Drawing for the job (mm, zero at the part's lowest x, y, z). Give positions to 0.01 mm unless a question says otherwise; leave off trailing zeros. Answer as a JSON object with one key per item and string values. Group by question number.
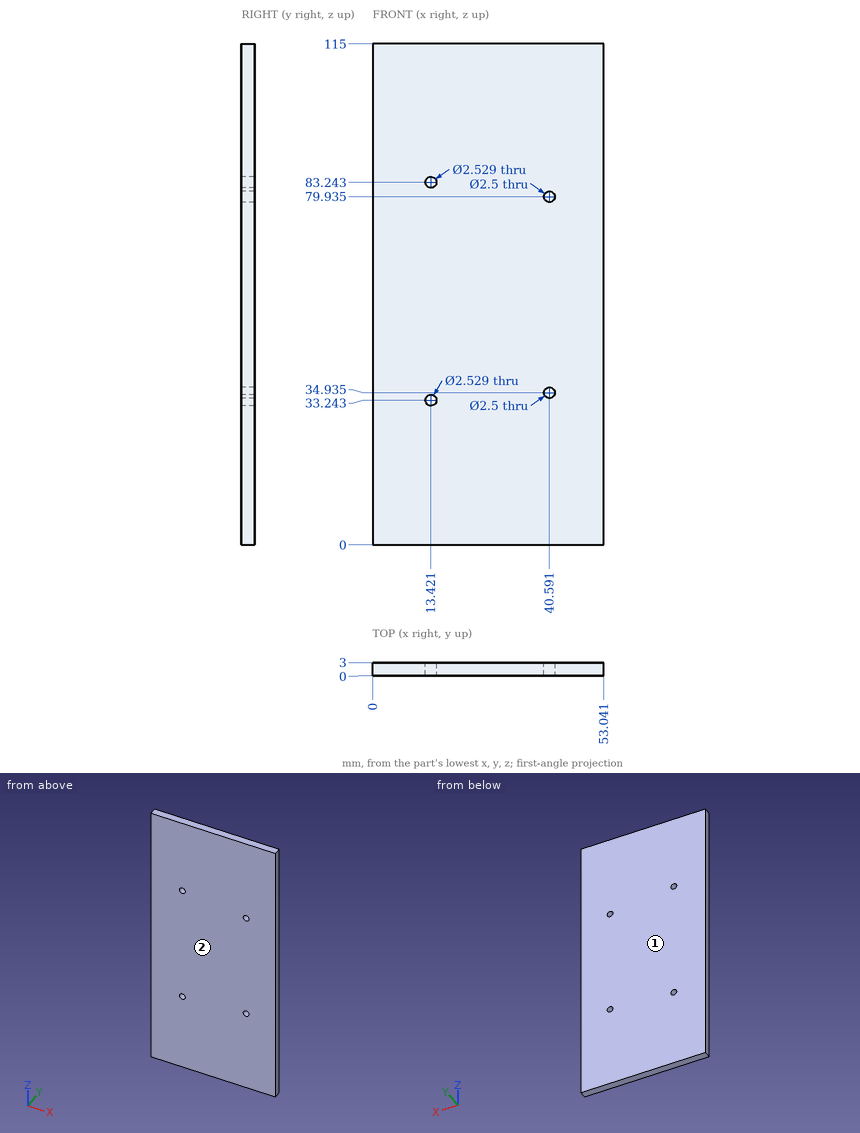
1) Mould opens along Y. For the marked faces 1 and 2 say: pulls with the +Y half, pulls with the -Y half, needs draft (parallel to the pull), parting line crosses it, or undercut.
2) Drop flat-ended pins along their axis: P1, Ø12, axis at x = 27.5, z = 63, coming from the -Y side; P2, Ø2, axis at x = 40.59, z = 34.93, coming from the -Y side. Give the stop position or say it passes through.
3) Probe line 1 (Z direction, x = 40, y = 1.55) (1 decimal); line 2 (Z direction, x = 14, y = 0.8); line 3 (X direction, y = 2.65, z = 81) (1 decimal). List the from-to ranges inside material, lowest first.
Verdict:
{
 "1": {"face 1": "pulls with the +Y half", "face 2": "pulls with the -Y half"},
 "2": {"P1": "y = 0", "P2": "through"},
 "3": {"line 1": "0 to 33.8, 36 to 78.8, 81 to 115", "line 2": "0 to 32.12, 34.37 to 82.12, 84.37 to 115", "line 3": "0 to 39.9, 41.2 to 53"}
}
